Autodesk Inventor part; units mm, degrees
ref_plane "YZ Plane" through (0, 0, 0) normal (1, 0, 0) x (0, 1, 0)
ref_plane "XZ Plane" through (0, 0, 0) normal (0, 1, 0) x (-1, 0, 0)
ref_plane "XY Plane" through (0, 0, 0) normal (0, 0, 1) x (1, 0, 0)
sketch "Sketch1" plane through (0, 0, 0) normal (0, 1, 0) x (-1, 0, 0)
  line L0 (0, 0) -> (25.4, 0)
  line L1 (25.4, 0) -> (25.4, -25.4)
  line L2 (25.4, -25.4) -> (0, -25.4)
  line L3 (0, -25.4) -> (0, 0)
  dimension "d0" = 25.4
  dimension "d1" = 25.4
extrude "Extrusion1" add sketch "Sketch1" along normal blind 450.85
sketch "Sketch2" plane through (0, 450.85, 0) normal (0, 1, 0) x (1, 0, 0)
  line L0 (-3.175, 3.175) -> (-22.225, 3.175)
  line L1 (-22.225, 3.175) -> (-22.225, 22.225)
  line L2 (-22.225, 22.225) -> (-3.175, 22.225)
  line L3 (-3.175, 22.225) -> (-3.175, 3.175)
  line L4 (0, 25.4) -> (-25.4, 25.4)
  line L5 (-25.4, 25.4) -> (-25.4, 0)
  line L6 (-25.4, 0) -> (0, 0)
  line L7 (0, 0) -> (0, 25.4)
  dimension "d4" = 3.175
  dimension "d5" = 3.175
  dimension "d6" = 3.175
  dimension "d7" = 3.175
extrude "Extrusion2" cut sketch "Sketch2" against normal blind 450.85 contours L0 L1 L2 L3
sketch "Sketch3" plane through (-25.4, 0, -25.4) normal (-1, 0, 0) x (0, 0, 1)
  circle A0 centre (12.7, 12.7) radius 1.4605
  line L0 (0, 0) -> (0, 450.85)
  line L1 (25.4, 0) -> (0, 0)
  circle A1 centre (12.7, 38.1) radius 1.4605
  circle A2 centre (12.7, 63.5) radius 1.4605
  circle A3 centre (12.7, 88.9) radius 1.4605
  circle A4 centre (12.7, 114.3) radius 1.4605
  circle A5 centre (12.7, 139.7) radius 1.4605
  circle A6 centre (12.7, 165.1) radius 1.4605
  circle A7 centre (12.7, 190.5) radius 1.4605
  circle A8 centre (12.7, 215.9) radius 1.4605
  circle A9 centre (12.7, 241.3) radius 1.4605
  circle A10 centre (12.7, 266.7) radius 1.4605
  circle A11 centre (12.7, 292.1) radius 1.4605
  circle A12 centre (12.7, 317.5) radius 1.4605
  circle A13 centre (12.7, 342.9) radius 1.4605
  circle A14 centre (12.7, 368.3) radius 1.4605
  circle A15 centre (12.7, 393.7) radius 1.4605
  circle A16 centre (12.7, 419.1) radius 1.4605
  circle A17 centre (12.7, 444.5) radius 1.4605
  dimension "d10" = 2.921
  dimension "d11" = 12.7
  dimension "d12" = 12.7
  dimension "d15" = 25.4
extrude "Extrusion3" cut sketch "Sketch3" against normal blind 25.4
equation "\"BendRadius\" = Thickness"
equation "\"BendReliefWidth\" = Thickness"
equation "\"BendReliefDepth\" = 0.5 * Thickness"
equation "\"CornerReliefSize\" = 4 * Thickness"
equation "\"MinimumRemnant\" = 2 * Thickness"
equation "\"TransitionRadius\" = BendRadius"
equation "\"JacobiRadiusSize\" = BendRadius"
equation "\"GapSize\" = Thickness"
properties part number "lil silver hangy thing"
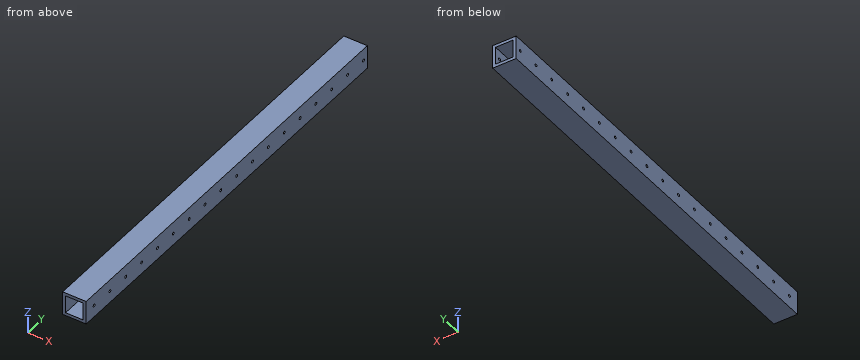
Geometry check sheet. Reference: the model listing, model coordinates, mm. Coordinates: 2 decimals unless noted, no trailing zeros. Loops run counter-clockwise (first coordinate to the right, second up) from the corner with the lowest first, then second, coordinate; pieces in that order, holes last.
Item 1: Sectioned sample at A-A, the plane x = -18. Record the boundary of the cut face in (y, z) (3 decimals).
Item 2: Thickness scan on line 1 (Z direction, x = -24.3, y = 292.1); line 2 (Z direction, x = -3.5, y = 149) (3 decimals). Record the ranges inside material, lowest first.
Item 3: Sectioned sample at B-B, the plane y = 96.5. Record the boundary of the cut face in (x, z) (3 decimals).
Item 4: Go/stop test with a flat-tipped pin: pin 1 Ø3.5 at (y, z) = (12.7, -12.7) entering from +X. Record where the tip stops, or that it passes through.
Check result:
1. outline: (0, -25.4) - (450.85, -25.4) - (450.85, -22.225) - (0, -22.225) - close; (0, -3.175) - (450.85, -3.175) - (450.85, 0) - (0, 0) - close
2. line 1: z = -25.4 to -14.16, -11.24 to 0
2. line 2: z = -25.4 to -22.225, -3.175 to 0
3. outline: (-25.4, -25.4) - (0, -25.4) - (0, 0) - (-25.4, 0) - close; hole (-22.225, -22.225) - (-3.175, -22.225) - (-3.175, -3.175) - (-22.225, -3.175) - close
4. pin 1: stops at x = 0
